Read the model definition and answer for the solid it produces. Units are mm, in the model's axes. A direction names the side the tool comes from. Give positions to 0.01 mm unless a question says otherwise; leave off trailing zeros. Order: outer loops, then holes, each group sorted by start corner. A loop starts at its lowest first (then second) coordinate and runs counter-clockwise, first axis right, second up. Notation, with made-up numbers: (-39, 34.25) -> (11, 34.25) arc R20 ccw to (11, 61.25) -> close; hole circle Ø4 at (43.5, 80.5). An arc over 180 degrees is marked (long way). Answer as CSV lines item,"result". Start each with the question number.
1) Find section B-B (y = -52.5). Determine the outline of the cut face in (x, z).
2) Find section C-C (x = 66.5). Determine the outline of the cut face in (y, z), and give its area (3 significant figures).
3) Flat-ended cylindrical pins translate along their axes: pin 1 Ø24 at (y, z) = (-58.5, 41.5) entering from -X; pin 2 Ø2 at (x, y) = (-49.5, -83) entering from +Z; pin 3 Ø15 at (y, z) = (-105.5, -19.5) entering from -X. Find the tip coordinate at first contact, or state that the pin passes through.
4) Straight lines are drawn through the part: L1, parallel to X at y = -86, z = -45; L2, parallel to Z at x = -57.5, y = -98; L3, parallel to Z at x = -10, y = -141.5. For each, find the intervals that lie inside material, in ascending order. Write a range as from..to.
5) Find section A-A (z = 46). Determine the outline of the cut face in (x, y).
6) The mould has two halves that part along Z. Classify faces 1 (the face through (-1, -74, -90)), 2 (the face through (65, -125, 51)), 3 (the face through (55, -74, 42)): +Z half, -Z half, draft (parallel to the pull), parting line (faces both ways), or undercut.
7) For faces 4 (the face through (65, -74, 42.174)), 5 (the face through (-53, -74, -65)), 6 (the face through (16, -74, 10)), determine the directions among +Z, -Z, +X, -X, +Y, -Y from which every point of the face is accessible in a straight line to the end or side of a thin tool.
8) Find section D-D (y = -133). Determine the outline of the cut face in (x, z).
```python
from build123d import *

# Parameters (mm, degrees)
F1_DEPTH = 150
F2_R     = 5
F3_DEPTH = 20.001
F4_W     = 100
F4_H     = 17.8262033769
F5_DEPTH = 20.001
F7_DEPTH = 25


with BuildPart() as f1:
    # F0 (on Front) → F1 (new body)
    with BuildSketch(Plane.XZ):
        Polygon((75, -90), (75, 90), (55, 90), (55, 10), (-25, 10), (-25, -40), (-75, -40), (-75, -90), align=None)
    extrude(amount=F1_DEPTH)

    # F2 (on face) → F3 (cut, through all)
    with BuildSketch(Plane(origin=(55, 0, 0), x_dir=(0, -1, 0), z_dir=(-1, 0, 0))):
        with Locations((75.9465023875, 69.8286518455)):
            Circle(F2_R)
    extrude(amount=-F3_DEPTH, mode=Mode.SUBTRACT)

    # F4 (on face) → F5 (cut, through all)
    with BuildSketch(Plane(origin=(55, 0, 0), x_dir=(0, -1, 0), z_dir=(-1, 0, 0))):
        with Locations((75, 51.0868983116)):
            Rectangle(F4_W, F4_H)
    extrude(amount=-F5_DEPTH, mode=Mode.SUBTRACT)

    # F6 (on face) → F7 (cut)
    with BuildSketch(Plane.XY.offset(-40)):
        with BuildLine():
            ThreePointArc((-42.7634136379, -115), (-52.7634136379, -105), (-62.7634136379, -115))
            Line((-62.7634136379, -115), (-42.7634136379, -115))
        make_face()
        with BuildLine():
            Line((-62.7634136379, -35), (-62.7634136379, -115))
            ThreePointArc((-62.7634136379, -115), (-52.7634136379, -105), (-42.7634136379, -115))
            Line((-42.7634136379, -115), (-42.7634136379, -35))
            ThreePointArc((-42.7634136379, -35), (-52.7634136379, -45), (-62.7634136379, -35))
        make_face()
        with BuildLine():
            Line((-42.7634136379, -115), (-62.7634136379, -115))
            ThreePointArc((-62.7634136379, -115), (-52.7634136379, -125), (-42.7634136379, -115))
        make_face()
        with BuildLine():
            ThreePointArc((-42.7634136379, -35), (-52.7634136379, -25), (-62.7634136379, -35))
            Line((-62.7634136379, -35), (-42.7634136379, -35))
        make_face()
        with BuildLine():
            Line((-42.7634136379, -35), (-62.7634136379, -35))
            ThreePointArc((-62.7634136379, -35), (-52.7634136379, -45), (-42.7634136379, -35))
        make_face()
    extrude(amount=-F7_DEPTH, mode=Mode.SUBTRACT)


solid = f1.part
```
Findings below:
1,outline,"(-75, -90) -> (75, -90) -> (75, 42.17) -> (55, 42.17) -> (55, 10) -> (-25, 10) -> (-25, -40) -> (-42.76, -40) -> (-42.76, -65) -> (-62.76, -65) -> (-62.76, -40) -> (-75, -40) -> close; (55, 60) -> (75, 60) -> (75, 90) -> (55, 90) -> close"
2,outline,"(-150, -90) -> (0, -90) -> (0, 90) -> (-150, 90) -> close; hole (-125, 42.17) -> (-25, 42.17) -> (-25, 60) -> (-125, 60) -> close; hole circle Ø10 at (-75.95, 69.83)"
2,area,"25,100 mm²"
3,pin 1,"x = 55"
3,pin 2,"z = -65"
3,pin 3,"x = -25"
4,L1,"-75..-62.76, -42.76..75"
4,L2,"-90..-65"
4,L3,"-90..10"
5,outline,"(55, -150) -> (75, -150) -> (75, -125) -> (55, -125) -> close; (55, -25) -> (75, -25) -> (75, 0) -> (55, 0) -> close"
6,face 1,"-Z half"
6,face 2,"undercut"
6,face 3,"draft"
7,face 4,"+X, -X"
7,face 5,"+Z"
7,face 6,"+Z, -X, +Y, -Y"
8,outline,"(-75, -90) -> (75, -90) -> (75, 90) -> (55, 90) -> (55, 10) -> (-25, 10) -> (-25, -40) -> (-75, -40) -> close"
